Verification items for this drawing (mm, ordinates from the low corner). A direction names the side the tool comes from. Give positions to 0.01 mm unless a question says otherwise; leave off trailing zeros. Order: outer loops, then holes, each group sorted by start corner. A loop starts at its lowest first (then second) coordinate and runs counter-clockwise, first axis right, second up. Notation, with made-up numbers: (28.25, 80) -> (60.25, 80) arc R12 ccw to (60.25, 98) -> close; hole circle Ø6 at (87, 63). An arc over 180 degrees is marked (long way). One line per question, with ' | ' between items.
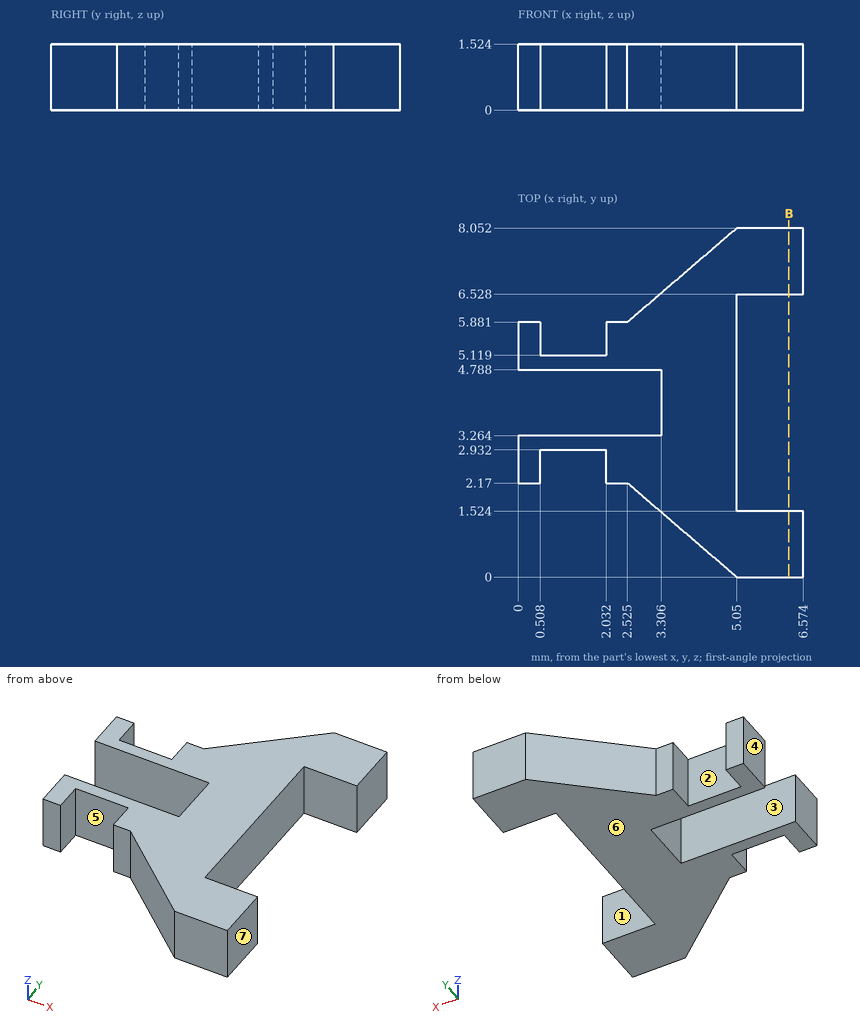
Q1. Section check B-B (x = 6.25). Enter the section's corners in (y, z) (1 decimal).
Result sheet:
outline: (0, 0) -> (1.5, 0) -> (1.5, 1.5) -> (0, 1.5) -> close; (6.5, 0) -> (8.1, 0) -> (8.1, 1.5) -> (6.5, 1.5) -> close
Q2. Thickness scan on line 1 (Y direction, x = 1, z = 0.7); line 2 (Y direction, x = 5.25, z = 0.7) (1 decimal); line 3 (X direction, y = 2.25, z = 0.5). Record the ranges inside material, lowest first.
Result sheet:
line 1: y = 2.93 to 3.26, 4.79 to 5.12 | line 2: y = 0 to 1.5, 6.5 to 8.1 | line 3: x = 0 to 0.51, 2.03 to 5.05
Q3. Access from +Z, -Z, +X, -X, +Y, -Y to the whole of each face (thin tool, end or side, straight path). Record for the marked faces 1, 2 and 3.
Result sheet:
face 1: +Z, -Z, +X | face 2: +Z, -Z, +Y | face 3: +Z, -Z, -X
Q4. Mould release check, pull along X, two halves, no side actions. Record for the marked faces 4, 5, 6 and 7: pulls with the +X half, pulls with the -X half, needs draft (parallel to the pull), parting line crosses it, or undercut.
Result sheet:
face 4: pulls with the -X half | face 5: undercut | face 6: needs draft | face 7: pulls with the +X half
Q5. Depth check by flat-ended pin: pin 1 Ø0.5 at (x, z) = (1.5, 1) entering from +Y; pin 2 Ø0.8 at (y, z) = (5.5, 1) entering from +X; pin 3 Ø0.5 at (x, z) = (2, 0.5) entering from -Y. Enter the tip coordinate at first touch or a pass-through.
Result sheet:
pin 1: stops at y = 5.12 | pin 2: stops at x = 5.05 | pin 3: stops at y = 2.17
